For this review, take the finished solid that the model builds, in its own axes (mm). Face numbers are marked on the shaded views. A direction names the side the tool comes from. Coordinates: 2 decimals unless noted, no trailing zeros. Write each loop counter-clockwise with the first axis right and the second up, starting at its lowest first coordinate (ties: lowest second). Pieces come first, ordered by that corner, then holes.
Autodesk Inventor part; units mm, degrees
ref_plane "YZ Plane" through (0, 0, 0) normal (1, 0, 0) x (0, 1, 0)
ref_plane "XZ Plane" through (0, 0, 0) normal (0, 1, 0) x (-1, 0, 0)
ref_plane "XY Plane" through (0, 0, 0) normal (0, 0, 1) x (1, 0, 0)
sketch "Sketch1" plane through (0, 0, 0) normal (0, 0, 1) x (1, 0, 0)
  line L0 (-26.4763, -7.5222) -> (152.9112, -7.5222)
  line L1 (-26.4763, -7.5222) -> (25.5399, 28.8999)
  line L2 (-26.4763, -7.5222) -> (37.0237, -7.5222) construction
  line L3 (25.5399, 28.8999) -> (152.9112, 28.8999)
  line L4 (152.9112, 28.8999) -> (152.9112, -7.5222)
  point P0 (0, 0)
  dimension "d0" = 179.3875
  dimension "d2" = 63.5
  dimension "d3" = 35
extrude "Extrusion1" add sketch "Sketch1" along normal blind 3.175
sketch "Sketch2" plane through (0, 0, 0) normal (0, 0, -1) x (-1, 0, 0)
  line L0 (-152.9112, -7.5222) -> (-152.9112, 28.8999)
  line L1 (-152.9112, 28.8999) -> (-25.5399, 28.8999)
  line L2 (-89.2255, 21.9149) -> (-70.1755, 21.9149)
  line L3 (-70.1755, 21.9149) -> (-70.1755, 18.7399)
  line L4 (-70.1755, 18.7399) -> (-108.2755, 18.7399)
  line L5 (-108.2755, 18.7399) -> (-108.2755, 21.9149)
  line L6 (-108.2755, 21.9149) -> (-89.2255, 21.9149)
  point P0 (0, 0)
  dimension "d7" = 19.05
  dimension "d8" = 3.175
  dimension "d9" = 38.1
  dimension "d10" = 3.175
extrude "Extrusion2" add sketch "Sketch2" along normal blind 79.2734
sketch "Sketch3" plane through (70.1755, 18.7399, 0) normal (0, -1, 0) x (1, 0, 0)
  line L0 (0, -79.2734) -> (19.05, -79.2734)
  line L1 (19.05, -79.2734) -> (19.05, -60.2234)
  line L2 (19.05, -60.2234) -> (0, -60.2234)
  line L3 (0, -60.2234) -> (0, -79.2734)
  point P0 (-70.1755, 0)
  dimension "d13" = 19.05
  dimension "d14" = 19.05
hole "Hole1" at (89.2255, 18.7399, -60.2234) direction (0, 1, 0) diameter 8.3312 end through all
properties part number "Left Forearm"
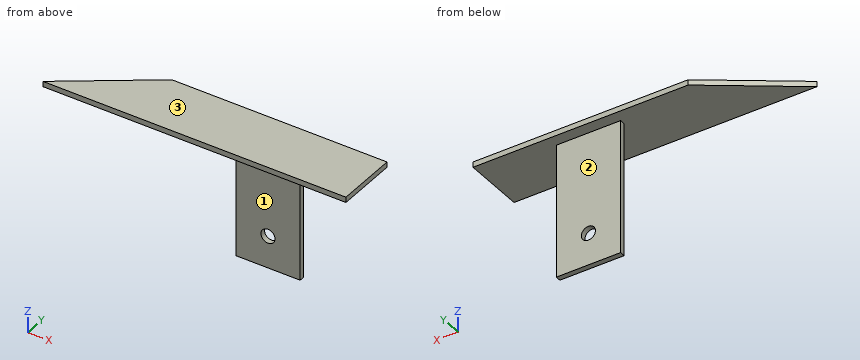
Q1. Add section A-A (z = -20.5). State the section outline as (x, y) points.
Ans:
outline: (70.18, 18.74) - (108.28, 18.74) - (108.28, 21.91) - (70.18, 21.91) - close
Q2. Tool access review of the marked faces 1, 2 and 3: name each direction out of +Z, -Z, +X, -X, +Y, -Y from which nothing blocks a thin tool from reaching the whole face with its end or side.
Ans:
face 1: -Z, +X, -X, -Y
face 2: -Z, +X, -X, +Y
face 3: +Z, +X, -X, +Y, -Y
Q3. Add section B-B (y = 5.5). State the section outline as (x, z) points (3 decimals).
Ans:
outline: (-7.879, 0) - (152.911, 0) - (152.911, 3.175) - (-7.879, 3.175) - close
Q4. For probe 1 along Z at (x, y) = (85.5, 13.5) (3 decimals); probe 2 along X at (y, z) = (20.5, -29); probe 3 along Y at (x, z) = (103, -7.5), list the stretches that pass through material, from the lowest coordinate up.
Ans:
probe 1: z = 0 to 3.175
probe 2: x = 70.18 to 108.28
probe 3: y = 18.74 to 21.91
Q5. Clearance check with flat-ended pins moving along their axes: pin 1 Ø12 at (y, z) = (24, -64.5) entering from -X; pin 2 Ø1.6 at (y, z) = (19.5, -45.5) entering from +X; pin 3 Ø11.5 at (x, z) = (93.5, -50) entering from +Y. State where each tip first meets the part, or that it passes through.
Ans:
pin 1: stops at x = 70.18
pin 2: stops at x = 108.28
pin 3: stops at y = 21.91
